Part model, mm, in its own coordinate system. Coordinates: 2 decimals unless noted, no trailing zeros. Loops run counter-clockwise (first coordinate to the right, second up) from the corner with the lowest first, then second, coordinate; pieces in that order, holes last. Notation, with made-up numbers: (58.5, 73) -> (113.5, 73) arc R19 cw to (113.5, 86) -> close; hole circle Ø9 at (-17, -16.75). An arc over 180 degrees is marked (long way). One line per question, with ' | ' between items. Start each with the question number.
1) Cut at A-A (x = 7.5). List the corners of the cut face in (y, z), plus the area to 3 significant figures.
2) Cut at C-C (z = 1.75). List the corners of the cut face in (x, y).
3) Probe L1, parallel to X at y = 41.5, z = 9.5; L2, parallel to Y at x = 6.75, z = 3; L3, parallel to Y at x = 7.75, z = 5. List the from-to ranges inside material, lowest first. Write a range as from..to.
4) Drop a flat-ended pin along its axis: pin 1 (1 mm diameter, centred on x = 8, z = 1.5, fed in from -Y). Give the stop position or say it passes through.
5) Cut at B-B (y = 42). List the corners of the cut face in (x, z).
from build123d import *

# Parameters (mm, degrees)
SKETCH_R         = 3.25
EXTRUDE023_DEPTH = 10
EXTRUDE022_DEPTH = 10


with BuildPart() as extrude023:
    # Sketch → Extrude023 (new body)
    with BuildSketch(Plane.XY):
        with Locations((6.505444, 43.780474)):
            Circle(SKETCH_R)
    extrude(amount=EXTRUDE023_DEPTH)


with BuildPart() as led_base:
    # Sketch → Extrude022 (new body)
    with BuildSketch(Plane.XY):
        with Locations((6.505444, 43.780474)):
            Circle(SKETCH_R)
    extrude(amount=EXTRUDE022_DEPTH)

    # Fusion010: union Extrude023
    add(extrude023.part)


solid = led_base.part
Reported:
1) outline: (40.69, 0) -> (46.87, 0) -> (46.87, 10) -> (40.69, 10) -> close | area: 61.9 mm²
2) outline: circle Ø6.5 at (6.51, 43.78)
3) L1: x = 4.19..8.82 | L2: y = 40.54..47.02 | L3: y = 40.78..46.78
4) pin 1: stops at y = 40.69
5) outline: (3.79, 0) -> (9.22, 0) -> (9.22, 10) -> (3.79, 10) -> close
